The model under review builds one solid part; all positions refer to its coordinate system, in mm. Give positions to 0.01 mm unless a question says otherwise; leave off trailing zeros. Order: outer loops, then holes, each group sorted by start corner. A loop starts at its lowest first (then second) coordinate and runs counter-clockwise, first axis right, second up. Notation, with made-up numbers: (64, 60) -> (74, 60) arc R4 cw to (74, 64) -> close; hole circle Ø1 at (-13.75, 19.5). An arc over 180 degrees is marked (long way). Answer as a JSON object with one key per item and string values. Group by question number.
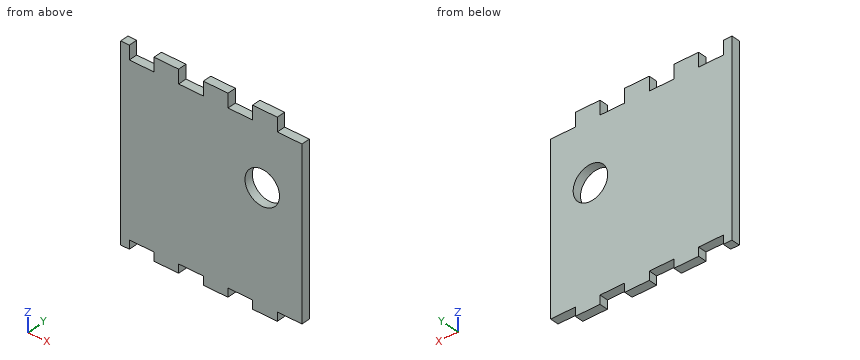
from build123d import *

# Parameters (mm, degrees)
F0_W     = 133.35
F0_H     = 139.7
F1_DEPTH = 6.35
F2_W     = 18.1428571429
F2_H     = 10.16
F2_H_2   = 6.35
F3_DEPTH = 25.4
F4_R     = 12.7
F5_DEPTH = 25.4


with BuildPart() as f1:
    # F0 (on Front) → F1 (new body)
    with BuildSketch(Plane.XZ):
        Rectangle(F0_W, F0_H)
    extrude(amount=F1_DEPTH)

    # F2 (on face) → F3 (cut)
    with BuildSketch(Plane.XZ.offset(6.35)):
        with Locations((57.6035714286, 64.77)):
            Rectangle(F2_W, F2_H)
        with Locations((-51.2535714286, 64.77)):
            Rectangle(F2_W, F2_H)
        with Locations((-14.9678571429, 64.77)):
            Rectangle(F2_W, F2_H)
        with Locations((21.3178571429, 64.77)):
            Rectangle(F2_W, F2_H)
        with Locations((-51.2535714286, -66.675)):
            Rectangle(F2_W, F2_H_2)
        with Locations((-14.9678571429, -66.675)):
            Rectangle(F2_W, F2_H_2)
        with Locations((21.3178571429, -66.675)):
            Rectangle(F2_W, F2_H_2)
        with Locations((57.6035714286, -66.675)):
            Rectangle(F2_W, F2_H_2)
    extrude(amount=-F3_DEPTH, mode=Mode.SUBTRACT)

    # F4 (on face) → F5 (cut)
    with BuildSketch(Plane.XZ.offset(6.35)):
        with Locations((37.465, 16.51)):
            Circle(F4_R)
    extrude(amount=-F5_DEPTH, mode=Mode.SUBTRACT)


solid = f1.part
1. For probe 1 along Z at (x, y) = (-20, -5); probe 2 along Z at (x, y) = (42, -3.25); probe 3 along X at (y, z) = (-2.5, 19) (1 decimal), list the stretches that pass through material, from the lowest coordinate up. Write a range as [from, to].
2. Take a section at D-D on x = -14.5. Give the boundary of the cut face in (y, z).
3. Take a section at C-C on x = 40. Give the boundary of the cut face in (y, z), plus the area to 3 significant figures.
4. Take a section at A-A on z = 16.51. Give the boundary of the cut face in (x, y) (3 decimals), plus the area to 3 significant figures.
5. For pin 1 (3 mm diameter, centred on x = -53, y = -4, fed in from +Z); pin 2 (1.9 mm diameter, centred on y = -4, z = 65.5, fed in from +X); pin 3 (1 mm diameter, centred on x = 21, y = -2, fed in from -Z); pin 4 (1.5 mm diameter, centred on x = -46, z = 49.5, fed in from +Y), all flat-tipped, find the tip position at first contact; note any pin that passes through.
Checks:
{
 "1": {"probe 1": "z = [-63.5, 59.69]", "probe 2": "z = [-69.85, 4.65], [28.37, 69.85]", "probe 3": "x = [-66.7, 25], [49.9, 66.7]"},
 "2": {"outline": "(-6.35, -63.5) -> (0, -63.5) -> (0, 59.69) -> (-6.35, 59.69) -> close"},
 "3": {"outline": "(-6.35, -69.85) -> (0, -69.85) -> (0, 4.07) -> (-6.35, 4.07) -> close; (-6.35, 28.95) -> (0, 28.95) -> (0, 69.85) -> (-6.35, 69.85) -> close", "area": "729 mm2"},
 "4": {"outline": "(-66.675, -6.35) -> (24.765, -6.35) -> (24.765, 0) -> (-66.675, 0) -> close; (50.165, -6.35) -> (66.675, -6.35) -> (66.675, 0) -> (50.165, 0) -> close", "area": "685 mm2"},
 "5": {"pin 1": "stops at z = 59.69", "pin 2": "stops at x = 48.53", "pin 3": "stops at z = -63.5", "pin 4": "stops at y = 0"}
}
